The drawing under review shows one solid part. Ordinate dimensions are in mm from its lowest x, y, z. A direction names the side the tool comes from. Give positions to 0.01 mm unless a question says otherwise; leave off trailing zeros. Order: outer loops, then holes, each group sorted by start corner. A loop starts at its lowest first (then second) coordinate and runs counter-clockwise, first axis right, second up. Notation, with made-up numbers: (80.25, 1.25) - (105.25, 1.25) arc R14 cw to (105.25, 21.25) - close; hole circle Ø7 at (53.5, 44). An arc over 180 degrees is marked (long way). Answer as a JSON object with one key per item and string values. Group by question number.
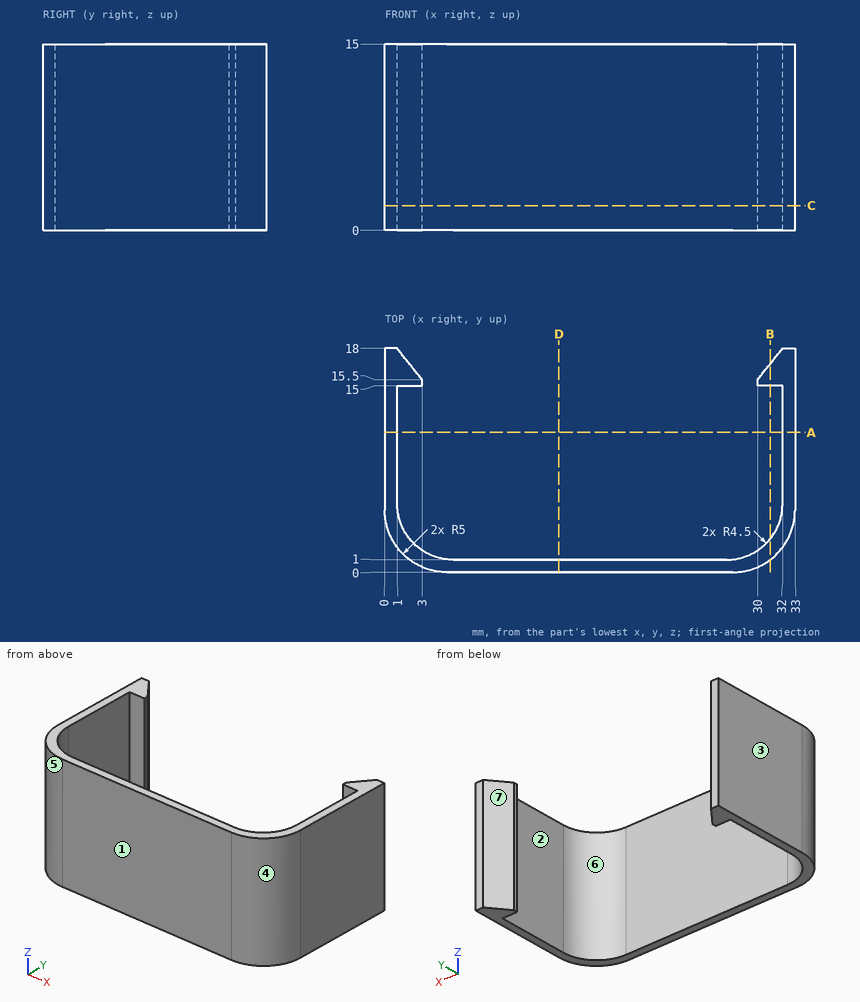
1) Consider section B-B (x = 31). Give the boundary of the cut face in (y, z).
2) Mouldability with a two-part tool opening along X and no side actions: class the marked faces 1, 2, 3 and 4 as released by +X, released by -X, zero draft, split by the parting line, or undercut.
3) For pin 1 (0.6 mm diameter, centred on x = 2, z = 10, fed in from -Y); pin 2 (0.6 mm diameter, centred on x = 31.5, z = 6, fed in from -Y); pin 3 (4.5 mm diameter, centred on x = 20.5, z = 4, fed in from +Y), all flat-tipped, find the tip position at first contact; note any pin that passes through.
4) For the marked faces 5, 6 and 7, list the 3-axis set-ups (+Z, -Z, +X, -X, +Y, -Y) from which the entire face can be reached by the end or side of a thin tool; tool diameter is ignored.
5) Consider section D-D (x = 14). Give the boundary of the cut face in (y, z), plus the area to 3 significant figures.
6) Consider section C-C (z = 2). Give the boundary of the cut face in (x, y).
7) For line 1 (X direction, y = 7, z = 2); line 2 (X direction, y = 15.25, z = 4); line 3 (Y direction, x = 23, z = 9), list the stretches that pass through material, from the lowest coordinate up.
8) Consider section A-A (y = 11.25). Give the boundary of the cut face in (x, z).
Result set:
{
 "1": {"outline": "(1, 0) - (2.67, 0) - (2.67, 15) - (1, 15) - close; (15, 0) - (16.75, 0) - (16.75, 15) - (15, 15) - close"},
 "2": {"face 1": "zero draft", "face 2": "undercut", "face 3": "released by -X", "face 4": "released by +X"},
 "3": {"pin 1": "stops at y = 0.79", "pin 2": "stops at y = 1.16", "pin 3": "stops at y = 1"},
 "4": {"face 5": "+Z, -Z, -X, -Y", "face 6": "+Z, -Z", "face 7": "+Z, -Z, +Y"},
 "5": {"outline": "(0, 0) - (1, 0) - (1, 15) - (0, 15) - close", "area": "15.0 mm2"},
 "6": {"outline": "(0, 5) arc R5 ccw to (5, 0) - (28, 0) arc R5 ccw to (33, 5) - (33, 18) - (32, 18) - (30, 15.5) - (30, 15) - (32, 15) - (32, 5.5) arc R4.5 cw to (27.5, 1) - (5.5, 1) arc R4.5 cw to (1, 5.5) - (1, 15) - (3, 15) - (3, 15.5) - (1, 18) - (0, 18) - close"},
 "7": {"line 1": "x = 0 to 1, 32 to 33", "line 2": "x = 0 to 3, 30 to 33", "line 3": "y = 0 to 1"},
 "8": {"outline": "(0, 0) - (1, 0) - (1, 15) - (0, 15) - close; (32, 0) - (33, 0) - (33, 15) - (32, 15) - close"}
}
